```python
from build123d import *

# Parameters (mm, degrees)
F1_DEPTH = 5


with BuildPart() as f1:
    # F0 (on Front) → F1 (new body)
    with BuildSketch(Plane.XZ):
        with BuildLine():
            Line((-29.8, -13.9), (29.8, -13.9))
            ThreePointArc((29.8, -13.9), (42.508398, -5.630864), (40.096296, 9.337895))
            ThreePointArc((40.096296, 9.337895), (39.135318, 10.896644), (38.8, 12.69685))
            Line((38.8, 12.69685), (38.8, 29.1))
            ThreePointArc((38.8, 29.1), (38.214214, 30.514214), (36.8, 31.1))
            Line((36.8, 31.1), (33.8, 31.1))
            ThreePointArc((33.8, 31.1), (33.092893, 30.807107), (32.8, 30.1))
            ThreePointArc((32.8, 30.1), (33.092893, 29.392893), (33.8, 29.1))
            Line((33.8, 29.1), (36.8, 29.1))
            Line((36.8, 29.1), (36.8, 26.3))
            Line((36.8, 26.3), (-36.8, 26.3))
            Line((-36.8, 26.3), (-36.8, 29.1))
            Line((-36.8, 29.1), (-33.8, 29.1))
            ThreePointArc((-33.8, 29.1), (-33.092893, 29.392893), (-32.8, 30.1))
            ThreePointArc((-32.8, 30.1), (-33.092893, 30.807107), (-33.8, 31.1))
            Line((-33.8, 31.1), (-36.8, 31.1))
            ThreePointArc((-36.8, 31.1), (-38.214214, 30.514214), (-38.8, 29.1))
            Line((-38.8, 29.1), (-38.8, 12.69685))
            ThreePointArc((-38.8, 12.69685), (-39.135318, 10.896644), (-40.096296, 9.337895))
            ThreePointArc((-40.096296, 9.337895), (-42.508398, -5.630864), (-29.8, -13.9))
        make_face()
        with BuildLine():
            ThreePointArc((29.8, 11.1), (40.9, 0), (29.8, -11.1))
            Line((29.8, -11.1), (-29.8, -11.1))
            ThreePointArc((-29.8, -11.1), (-40.9, 0), (-29.8, 11.1))
            Line((-29.8, 11.1), (29.8, 11.1))
        make_face(mode=Mode.SUBTRACT)
        with BuildLine():
            ThreePointArc((-31, 13.7), (-36, 18.7), (-31, 23.7))
            Line((-31, 23.7), (31, 23.7))
            ThreePointArc((31, 23.7), (36, 18.7), (31, 13.7))
            Line((31, 13.7), (-31, 13.7))
        make_face(mode=Mode.SUBTRACT)
    extrude(amount=F1_DEPTH)


solid = f1.part
```
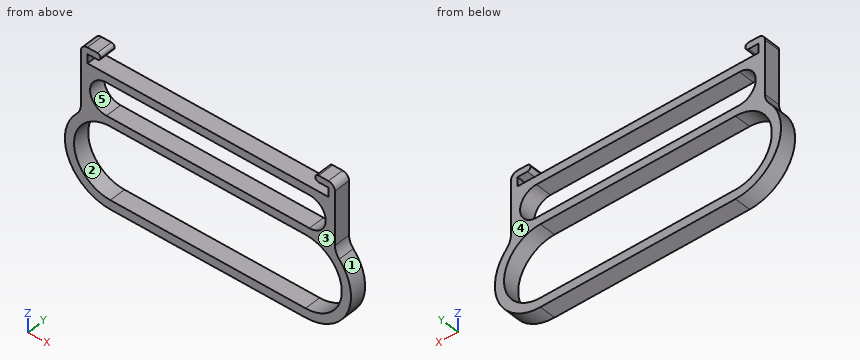
Geometry check sheet. Reference: the model listing, model coordinates, mm. Face numbers are marked on the shaded views. A direction names the side the tool comes from. Round coordinates to 2 decimals unless told otherwise and drop trailing zeros. Loops run counter-clockwise (first coordinate to the right, second up) from the corner with the lowest first, then second, coordinate; pieces in that order, holes last. Notation, with made-up numbers: (9.25, 8) - (48.25, 8) arc R26 cw to (48.25, 35) - close; hole circle Ø7 at (-30.75, 66.25). An arc over 180 degrees is marked (long way). Write item = value, one per line. Start each with the question number.
1. Section check B-B on y = -2. Enter the section's corners in (x, z).
2. Set-up check for the marked faces 4 and 5: record each of +Z, -Z, +X, -X, +Y, -Y from which the full face is reachable in a straight line by a thin tool's end or side.
3. Section check C-C on x = -26.5. Enter the section's corners in (y, z).
4. Section check A-A on z = 0. Enter the section's corners in (x, y), then the cut area to 3 significant figures.
5. Mould release check, pull along Z, two halves, no side actions. Record for the marked faces 1, 2 and 3: released by +Z, released by -Z, zero draft, split by the parting line, or undercut.
6. Depth check by flat-ended pin: pin 1 (3 mm diameter, centred on x = -28, y = -1, fed in from +Z); pin 2 (1.4 mm diameter, centred on y = -2.5, z = 28, fed in from -X); pin 3 (1.5 mm diameter, centred on x = -36, y = -3.5, fed in from -Z); pin 4 (2 mm diameter, centred on y = -2.5, z = -0.5, fed in from +X). Enter the tip coordinate at first touch or a pass-through.
7. Section check D-D on z = 22. Enter the section's corners in (x, y), then the cut area to 3 significant figures.
8. Thickness scan on line 1 (Z direction, x = -4.5, y = -1.4); line 2 (X direction, y = -1.4, z = 0); line 3 (X direction, y = -4.1, z = 29). Record the ranges inside material, lowest first.
Working result:
q1.outline = (-40.1, 9.34) arc R13.9 ccw to (-29.8, -13.9) - (29.8, -13.9) arc R13.9 ccw to (40.1, 9.34) arc R5 cw to (38.8, 12.7) - (38.8, 29.1) arc R2 ccw to (36.8, 31.1) - (33.8, 31.1) arc R1 ccw to (32.8, 30.1) arc R1 ccw to (33.8, 29.1) - (36.8, 29.1) - (36.8, 26.3) - (-36.8, 26.3) - (-36.8, 29.1) - (-33.8, 29.1) arc R1 ccw to (-32.8, 30.1) arc R1 ccw to (-33.8, 31.1) - (-36.8, 31.1) arc R2 ccw to (-38.8, 29.1) - (-38.8, 12.7) arc R5 cw to start; hole (-31, 13.7) - (31, 13.7) arc R5 ccw to (31, 23.7) - (-31, 23.7) arc R5 ccw to start; hole (-29.8, -11.1) - (29.8, -11.1) arc R11.1 ccw to (29.8, 11.1) - (-29.8, 11.1) arc R11.1 ccw to start
q2.face_4 = +Z, -Z, +X, -X, +Y
q2.face_5 = +Y, -Y
q3.outline = (-5, -13.9) - (0, -13.9) - (0, -11.1) - (-5, -11.1) - close; (-5, 11.1) - (0, 11.1) - (0, 13.7) - (-5, 13.7) - close; (-5, 23.7) - (0, 23.7) - (0, 26.3) - (-5, 26.3) - close
q4.outline = (-43.7, -5) - (-40.9, -5) - (-40.9, 0) - (-43.7, 0) - close; (40.9, -5) - (43.7, -5) - (43.7, 0) - (40.9, 0) - close
q4.area = 28.0 mm^2
q5.face_1 = split by the parting line
q5.face_2 = undercut
q5.face_3 = zero draft
q6.pin_1 = 26.3
q6.pin_2 = -38.8
q6.pin_3 = -12.79
q6.pin_4 = 43.7
q7.outline = (-38.8, -5) - (-34.76, -5) - (-34.76, 0) - (-38.8, 0) - close; (34.76, -5) - (38.8, -5) - (38.8, 0) - (34.76, 0) - close
q7.area = 40.4 mm^2
q8.line_1 = -13.9 to -11.1, 11.1 to 13.7, 23.7 to 26.3
q8.line_2 = -43.7 to -40.9, 40.9 to 43.7
q8.line_3 = -38.8 to -36.8, 36.8 to 38.8
